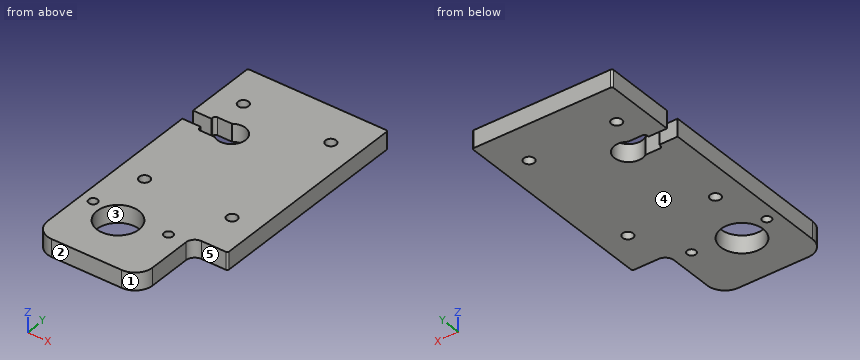
```python
from build123d import *

# Parameters (mm, degrees)
SKETCH_R    = 3
SKETCH_R_2  = 2.5
SKETCH_R_3  = 12
PAD_DEPTH   = 10
FILLET_R    = 1
FILLET001_R = 5
FILLET002_R = 10
FILLET003_R = 1.6


with BuildPart() as part:
    # Sketch → Pad (new body)
    with BuildSketch(Plane.XY):
        with BuildLine():
            Line((-25, 45), (55, 45))
            Line((55, 45), (55, -75))
            Line((35, -75), (55, -75))
            Line((35, -115), (35, -75))
            Line((-25, -115), (35, -115))
            Line((-25, -4), (-25, -115))
            Line((-14.5, -4), (-25, -4))
            Line((-14.5, -6.5), (-14.5, -4))
            Line((-14.5, -6.5), (-4.66369, -6.5))
            ThreePointArc((-4.66369, -6.5), (8, 0), (-4.66369, 6.5))
            Line((-14.5, 6.5), (-4.66369, 6.5))
            Line((-14.5, 6.5), (-14.5, 4))
            Line((-14.5, 4), (-25, 4))
            Line((-25, 45), (-25, 4))
        make_face()
        with Locations((-10, -52)):
            Circle(SKETCH_R, mode=Mode.SUBTRACT)
        with Locations((40, -52)):
            Circle(SKETCH_R, mode=Mode.SUBTRACT)
        with Locations((40, 22)):
            Circle(SKETCH_R, mode=Mode.SUBTRACT)
        with Locations((-10, 22)):
            Circle(SKETCH_R, mode=Mode.SUBTRACT)
        with Locations((25, -80)):
            Circle(SKETCH_R_2, mode=Mode.SUBTRACT)
        with Locations((-18, -80)):
            Circle(SKETCH_R_2, mode=Mode.SUBTRACT)
        with Locations((0, -85)):
            Circle(SKETCH_R_3, mode=Mode.SUBTRACT)
    extrude(amount=PAD_DEPTH)

    # Fillet
    fillet_edges = [part.edges().sort_by_distance(p)[0] for p in [
        (55, -75, 5),
        (55, 45, 5),
        (-25, 45, 5),
    ]]
    fillet(fillet_edges, radius=FILLET_R)

    # Fillet001
    fillet001_edges = [part.edges().sort_by_distance(p)[0] for p in [
        (35, -75, 5),
    ]]
    fillet(fillet001_edges, radius=FILLET001_R)

    # Fillet002
    fillet002_edges = [part.edges().sort_by_distance(p)[0] for p in [
        (35, -115, 5),
        (-25, -115, 5),
    ]]
    fillet(fillet002_edges, radius=FILLET002_R)

    # Fillet003
    fillet003_edges = [part.edges().sort_by_distance(p)[0] for p in [
        (-14.5, 6.5, 5),
        (-14.5, -6.5, 5),
    ]]
    fillet(fillet003_edges, radius=FILLET003_R)


solid = part.part
```
Source: CAD feature listing. Evaluate the final solid. Frame: model axes, mm. Face numbers are marked on the shaded views. A direction names the side the tool comes from. Give positions to 0.01 mm unless a question says otherwise; leave off trailing zeros. Write each loop counter-clockwise with the first axis right and the second up, starting at its lowest first coordinate (ties: lowest second). Pieces come first, ordered by that corner, then holes.
1. Pull-direction query (X, two-part tool) for the marked faces 1, 2 and 3; classes: +X half, -X half, draft (parallel to the pull), parting line (faces both ways), or undercut.
2. Section query A-A (y = -52). Return the cut outline in (x, z), then the cut area to 3 significant figures.
3. Material intervals for line 1 along Y through (x, z) = (40, 3.5); line 2 along Y through (x, z) = (3.5, 5.25); line 3 along Y through (x, z) = (-10, 5.25), sorted ascending.
4. Section query B-B (y = -85). Return the cut outline in (x, z).
5. First-contact query: pin 1 (1.5 mm diameter, centred on x = 27, z = 6.5, fed in from -Y); pin 2 (3 mm diameter, centred on x = -20, z = 3, fed in from -Y); pin 3 (2 mm diameter, centred on x = 40.5, z = 2.5, fed in from -Y). Flat tips, straight axial feed; report the tip coordinate or a pass-through.
6. Section query C-C (z = 3.5). Count the separate pieces of the cut face and the enclosed holes in it, then the cut area to 3 significant figures.
7. Section query D-D (x = -18). Return the cut outline in (y, z).
8. Access query for the marked faces 4 and 5. Directions: +Z, -Z, +X, -X, +Y, -Y. A direction counts if a zero-diameter tool reaches every point of the face in a straight line with its end or side. Return the directions, or none.
Output values:
1. face 1: +X half
1. face 2: draft
1. face 3: undercut
2. outline: (-25, 0) - (-13, 0) - (-13, 10) - (-25, 10) - close; (-7, 0) - (37, 0) - (37, 10) - (-7, 10) - close; (43, 0) - (55, 0) - (55, 10) - (43, 10) - close
2. area: 680 mm2
3. line 1: y = -75 to -55, -49 to 19, 25 to 45
3. line 2: y = -115 to -96.48, -73.52 to -7.19, 7.19 to 45
3. line 3: y = -115 to -91.63, -78.37 to -55, -49 to -6.5, 6.5 to 19, 25 to 45
4. outline: (-25, 0) - (-12, 0) - (-12, 10) - (-25, 10) - close; (12, 0) - (35, 0) - (35, 10) - (12, 10) - close
5. pin 1: stops at y = -114.92
5. pin 2: stops at y = -114.37
5. pin 3: stops at y = -75.03
6. separate pieces: 1
6. enclosed holes: 7
6. area: 11,000 mm2
7. outline: (-114.54, 0) - (-82.5, 0) - (-82.5, 10) - (-114.54, 10) - close; (-77.5, 0) - (-4, 0) - (-4, 10) - (-77.5, 10) - close; (4, 0) - (45, 0) - (45, 10) - (4, 10) - close
8. face 4: -Z, +X, -X, +Y, -Y
8. face 5: +Z, -Z, +X, -Y
